The listing builds one solid part. Answer for the finished solid, in the listing's coordinates (mm). A direction names the side the tool comes from. Round coordinates to 2 decimals unless told otherwise and drop trailing zeros. Write each loop counter-clockwise with the first axis right and the second up, starting at its lowest first coordinate (ties: lowest second). Pieces come first, ordered by that corner, then holes.
Item 1: Find section D-D on x = 14.5. Give the vertices of the cut face in (y, z), then the cut area to 3 significant figures.
Item 2: Find section B-B on z = 3.25. Give the number of separate pieces and of enclosed holes in the cut face, then the cut area to 3 significant figures.
Item 3: Find the intervals of material crossed by probe 1 along Y at (x, z) = (-4, 5.5); probe 2 along Y at (x, z) = (19, 7.75); probe 3 along Y at (x, z) = (-6, 11), in increasing order.
Item 4: A tool of negligible diameter and unlimited length cuts with its end or side. For faces 1 (the face through (7.605, 30.268, 12.197)), 2 (the face through (17, 5, 16)), 3 (the face through (-3, 17.8, 6)), 4 (the face through (18, 10, 6)), 5 (the face through (18, 17.8, 6)), from which of +Z, -Z, +X, -X, +Y, -Y can it reach the whole face along a straight path? Write none if from no direction.
Item 5: Find section C-C on y = 46.5. Give the vertices of the cut face in (x, z).
Item 6: Each of these flat-tipped pins is pushed along its axis until it touches: pin 1 (5 mm diameter, centred on x = 19, z = 7.5, fed in from -Y); pin 2 (2 mm diameter, centred on x = -2.5, z = 15, fed in from +Y); pin 3 (6 mm diameter, centred on x = 18.5, y = 15.5, fed in from +Z). Where does it stop, or does it pass through?
Item 7: For a pull along X with two mould halves and no side action, classify faces 6 (the face through (-3.82, 48.39, 5.92)), 7 (the face through (-3, 2, 12)), 8 (the face through (22.43, 2.54, 12.6)) as +X half, -X half, draft (parallel to the pull), parting line (faces both ways), or undercut.
Item 8: Find section A-A on x = 19. Give the vertices of the cut face in (y, z), then the cut area to 3 significant figures.
Autodesk Inventor part; units mm, degrees
ref_plane "Work Plane1" through (0, 0, 0) normal (0, -1, 0) x (1, 0, 0)
ref_plane "YZ Plane" through (0, 0, 0) normal (1, 0, 0) x (0, 1, 0)
ref_plane "XZ Plane" through (0, 0, 0) normal (0, 1, 0) x (-1, 0, 0)
sketch "Sketch1" plane through (0, 0, 0) normal (0, 0, 1) x (1, 0, 0)
  line L0 (0, 0) -> (15, 0)
  line L1 (15, 0) -> (15, 50)
  line L2 (15, 50) -> (0, 50)
  line L3 (0, 50) -> (0, 0)
  dimension "d0" = 15
  dimension "d1" = 50
extrude "Extrusion1" add sketch "Sketch1" along normal blind 20
sketch "Sketch2" plane through (15, 0, 0) normal (1, 0, 0) x (0, 0, -1)
  circle A0 centre (0, 30) radius 12.2
  line L0 (0, 50) -> (-20, 50)
  line L1 (0, 0) -> (0, 50)
  line L2 (0, 50) -> (0, 0)
  line L3 (-20, 0) -> (-20, 50)
  point P0 (0, 17.8)
  point P1 (0, 42.2)
  dimension "d4" = 24.4
  dimension "d5" = 20
  dimension "d6" = 20
extrude "Extrusion2" cut sketch "Sketch2" against normal through all contours L1 A0 picked at (-4.6431, 33.0439)
sketch "Sketch3" plane through (15, 0, 20) normal (1, 0, 0) x (0, 0, -1)
  line L0 (20, 50) -> (0, 50)
  line L1 (20, 50) -> (8, 50)
  line L2 (8, 50) -> (8, 42.2)
  line L3 (8, 42.2) -> (20, 42.2)
  line L4 (20, 42.2) -> (20, 50)
  line L5 (-6.7049, 30) -> (32.7164, 30)
  line L6 (20, 10) -> (0, 10)
  line L7 (8, 10) -> (8, 17.8)
  line L8 (8, 17.8) -> (20, 17.8)
  line L9 (20, 17.8) -> (20, 10)
  point P0 (20, 0)
  dimension "d9" = 12
  dimension "d10" = 7.8
  dimension "d11" = 20
extrude "Extrusion3" add sketch "Sketch3" along normal blind 8
sketch "Sketch4" plane through (0, 0, 0) normal (0, 0, -1) x (-1, 0, 0)
  circle A0 centre (-19, 46.5) radius 1.4
  line L0 (0, 50) -> (-23, 50)
  line L1 (-23, 42.2) -> (-23, 50)
  circle A1 centre (-19, 14.3) radius 1.4
  line L2 (-15, 17.8) -> (-23, 17.8)
  line L3 (-23, 10) -> (-23, 17.8)
  point P0 (0, 0)
  dimension "d14" = 2.8
  dimension "d15" = 3.5
  dimension "d16" = 4
  dimension "d17" = 2.8
  dimension "d18" = 3.5
  dimension "d43" = 4
extrude "Extrusion4" cut sketch "Sketch4" against normal through all
sketch "Sketch5" plane through (0, 0, 20) normal (-1, 0, 0) x (0, 0, 1)
  line L0 (-20, 42.2) -> (-20, 50)
  line L1 (-8, 42.2) -> (-20, 42.2)
  line L2 (-20, 50) -> (-8, 50)
  line L3 (-8, 50) -> (-8, 42.2)
  line L4 (-8, 42.2) -> (-20, 42.2)
  line L5 (-20, 42.2) -> (-20, 50)
  arc A0 (-20, 17.8) -> (-20, 42.2) centre (-20, 30) ccw
  line L6 (-8, 10) -> (-20, 10)
  line L7 (-20, 17.8) -> (-8, 17.8)
  line L8 (-8, 17.8) -> (-8, 10)
  line L9 (-8, 10) -> (-20, 10)
  line L10 (-20, 10) -> (-20, 17.8)
  point P0 (-20, 0)
extrude "Extrusion5" add sketch "Sketch5" along normal blind 8
sketch "Sketch6" plane through (0, 0, 0) normal (0, 0, -1) x (-1, 0, 0)
  circle A0 centre (4, 47) radius 1.4
  line L0 (8, 50) -> (8, 42.2)
  line L1 (8, 50) -> (-23, 50)
  circle A1 centre (4, 14.8) radius 1.4
  line L2 (0, 17.8) -> (8, 17.8)
  line L3 (8, 17.8) -> (8, 10)
  point P0 (0, 0)
  point P1 (8, 46.1)
  dimension "d23" = 2.8
  dimension "d24" = 4
  dimension "d25" = 3
  dimension "d26" = 2.8
  dimension "d27" = 3
  dimension "d44" = 4
extrude "Extrusion6" cut sketch "Sketch6" against normal through all
ref_plane "Work Plane1" through (0, 0, 0) normal (0, -1, 0) x (1, 0, 0)
sketch "Sketch7" plane through (0, 0, 0) normal (0, -1, 0) x (1, 0, 0)
  line L0 (0, 0) -> (0, 20)
  line L1 (0, 20) -> (-8, 20)
  line L2 (-8, 20) -> (-8, 12)
  line L3 (-8, 12) -> (0, 12)
  line L4 (0, 12) -> (0, 20)
  line L5 (0, 0) -> (15, 0)
  line L6 (7.5, 0) -> (7.5, 20)
  line L7 (15, 20) -> (0, 20)
  circle A0 centre (-4, 16) radius 1.4
  line L8 (15, 0) -> (15, 20)
  line L9 (15, 20) -> (23, 20)
  line L10 (23, 20) -> (23, 12)
  line L11 (23, 12) -> (15, 12)
  circle A1 centre (19, 16) radius 1.4
  dimension "d30" = 8
  dimension "d31" = 8
  dimension "d32" = 2.8
  dimension "d41" = 4
extrude "Extrusion7" add sketch "Sketch7" against normal blind 5 contours L3 L2 L1 L0 | L8 L9 L10 L11
fillet "Fillet1" radius 2 2 edges at (23, 2.5, 20) (23, 2.5, 12)
fillet "Fillet2" radius 2 2 edges at (-8, 2.5, 12) (-8, 2.5, 20)
fillet "Fillet3" radius 2 2 edges at (23, 17.8, 6) (23, 10, 6)
fillet "Fillet4" radius 2 2 edges at (-8, 10, 6) (-8, 17.8, 6)
fillet "Fillet5" radius 2 2 edges at (-8, 50, 6) (-8, 42.2, 6)
fillet "Fillet6" radius 2 2 edges at (23, 50, 6) (23, 42.2, 6)
sketch "Sketch8" plane through (15, 10, 12) normal (0, 0, 1) x (1, 0, 0)
  point P0 (-15, -10)
sketch "Sketch9" plane through (0, 5, 0) normal (0, 1, 0) x (1, 0, 0)
  point P0 (0, 0)
sketch "Sketch10" plane through (15, 10, 12) normal (0, 0, 1) x (1, 0, 0)
  point P0 (-15, -10)
sketch "Sketch11" plane through (0, 42.2, 12) normal (0, 0, 1) x (1, 0, 0)
  point P0 (0, -42.2)
sketch "Sketch12" plane through (15, 42.2, 12) normal (0, 0, 1) x (1, 0, 0)
  point P0 (-15, -42.2)
sketch "Sketch13" plane through (0, 42.2, 12) normal (0, 0, 1) x (1, 0, 0)
  point P0 (0, -42.2)
properties part number "üst döner blok"
Check values:
1. outline: (0, 0) - (17.8, 0) arc R12.2 cw to (42.2, 0) - (50, 0) - (50, 20) - (0, 20) - close
1. area: 766 mm2
2. separate pieces: 2
2. enclosed holes: 4
2. area: 615 mm2
3. probe 1: y = 10 to 13.4, 16.2 to 17.8, 42.2 to 45.6, 48.4 to 50
3. probe 2: y = 10 to 12.9, 15.7 to 17.8, 42.2 to 45.1, 47.9 to 50
3. probe 3: y = 10 to 17.8, 42.2 to 50
4. face 1: -Z, +X, -X
4. face 2: +Z, -Z, +X, +Y
4. face 3: +Z, -Z, -X
4. face 4: +Z, -Z, +X, -Y
4. face 5: +Z, -Z, +X
5. outline: (-8, 0) - (-5.31, 0) - (-5.31, 12) - (-8, 12) - close; (-2.69, 0) - (17.6, 0) - (17.6, 12) - (15, 12) - (15, 20) - (0, 20) - (0, 12) - (-2.69, 12) - close; (20.4, 0) - (23, 0) - (23, 12) - (20.4, 12) - close
6. pin 1: stops at y = 10
6. pin 2: stops at y = 5
6. pin 3: stops at z = 12
7. face 6: undercut
7. face 7: draft
7. face 8: +X half
8. outline: (0, 12) - (5, 12) - (5, 14.6) - (0, 14.6) - close; (0, 17.4) - (5, 17.4) - (5, 20) - (0, 20) - close; (10, 0) - (12.9, 0) - (12.9, 12) - (10, 12) - close; (15.7, 0) - (17.8, 0) - (17.8, 12) - (15.7, 12) - close; (42.2, 0) - (45.1, 0) - (45.1, 12) - (42.2, 12) - close; (47.9, 0) - (50, 0) - (50, 12) - (47.9, 12) - close
8. area: 146 mm2
